Autodesk Inventor part; units mm, degrees
ref_plane "YZ Plane" through (0, 0, 0) normal (1, 0, 0) x (0, 1, 0)
ref_plane "XZ Plane" through (0, 0, 0) normal (0, 1, 0) x (-1, 0, 0)
ref_plane "XY Plane" through (0, 0, 0) normal (0, 0, 1) x (1, 0, 0)
sketch "Skizze1" plane through (0, 0, 0) normal (0, 1, 0) x (-1, 0, 0)
  line L0 (2.5, -1.4434) -> (0, -2.8868)
  line L1 (0, -2.8868) -> (-2.5, -1.4434)
  line L2 (-2.5, -1.4434) -> (-2.5, 1.4434)
  line L3 (-2.5, 1.4434) -> (0, 2.8868)
  line L4 (0, 2.8868) -> (2.5, 1.4434)
  line L5 (2.5, 1.4434) -> (2.5, -1.4434)
  point P0 (0, 0)
  point P1 (0, 0)
  point P2 (0, 0)
  dimension "d0" = 5
extrude "Extrusion1" add sketch "Skizze1" against normal blind 17
hole "Bohrung1" at (0, 0, 0) direction (0, -1, 0) diameter 2.013 depth 8 tip angle 118
sketch "Skizze2" plane through (0, -17, 0) normal (0, -1, 0) x (1, 0, 0)
  circle A0 centre (0, 0) radius 1.0065
  circle A1 centre (0, 0) radius 1.25
  dimension "d10" = 2.5
extrude "Extrusion2" add sketch "Skizze2" along normal blind 6 contours A0 | A1
thread "Gewinde1"
chamfer "Fasen1" distance 0.25 angle 45 1 edges at (-1.25, -23, 0)
chamfer "Fasen2" distance 0.3 angle 45 12 edges at (2.5, 0, 0) (1.25, 0, 2.1651) (-1.25, 0, 2.1651) (-2.5, 0, 0) (-1.25, 0, -2.1651) (1.25, 0, -2.1651) (2.5, -17, 0) (1.25, -17, 2.1651) (-1.25, -17, 2.1651) (-2.5, -17, 0) (-1.25, -17, -2.1651) (1.25, -17, -2.1651)
properties part number "Abstandsbolzen 17mm"
Work out the finished part from the listing and answer in its coordinate system (mm). A direction names the side the tool comes from. Give positions to 0.01 mm unless a question says otherwise; leave off trailing zeros. Loops run counter-clockwise (first coordinate to the right, second up) from the corner with the lowest first, then second, coordinate; pieces in that order, holes last. Notation, with made-up numbers: (11.25, 35) - (51.25, 35) arc R17 cw to (51.25, 66) - close; hole circle Ø8 at (14.25, 19.5). An arc over 180 degrees is marked (long way). Use CSV: the item, a comma, the result in double quotes. Start each with the question number.
(1) Find section D-D, the plane z = 2.3. Determine the outline of the cut face in (x, y).
(2) A tool of negligible diameter and unlimited length cuts with its end or side. For faces 5 (the face through (1, 0, -1)), 6 (the face through (-0.27, -19.83, 1.22)), from which of +Z, -Z, +X, -X, +Y, -Y can it reach the whole face along a straight path? Write none if from no direction.
(3) Find the intervals of material crossed by L1, parallel to X at y = -4.5, z = 0; L2, parallel to Y at x = 0.7, z = 1.6; L3, parallel to X at y = -2.75, z = 0.35, in increasing order.
(4) Find section B-B, the plane y = -10. Determine the outline of the cut face in (x, z), plus the area to 3 significant figures.
(5) Determine the mould class of faces 1 (the face through (1.233, -8.385, -2.175)), 2 (the face through (0.05, -8.5, 0.17)), 3 (the face through (-1.191, -0.148, -2.023)), 4 (the face through (1, -17, 1)) for opening direction X: released by +X, released by -X, zero draft, split by the parting line, or undercut.
(6) Each of these flat-tipped pins is pushed along its axis until it touches: pin 1 (1 mm diameter, centred on x = 1, y = -7, fed in from +Z); pin 2 (2 mm diameter, centred on x = -0.5, y = -10, fed in from -Z); pin 3 (3 mm diameter, centred on x = 2, y = -3.5, fed in from -Z). Where does it stop, or does it pass through?
(7) Find section A-A, the plane y = -2.5. Determine the outline of the cut face in (x, z), plus the area to 3 significant figures.
(8) Find section C-C, the plane x = -1.45. Determine the outline of the cut face in (y, z).
Results found:
1,outline,"(-1.02, -16.7) - (-0.42, -17) - (0.42, -17) - (1.02, -16.7) - (1.02, -0.3) - (0.42, 0) - (-0.42, 0) - (-1.02, -0.3) - close"
2,face 5,"+Z, -Z, +X, -X, +Y"
2,face 6,"-Y"
3,L1,"-2.5 to -1.01, 1.01 to 2.5"
3,L2,"-17 to 0"
3,L3,"-2.5 to -0.94, 0.94 to 2.5"
4,outline,"(-2.5, -1.44) - (0, -2.89) - (2.5, -1.44) - (2.5, 1.44) - (0, 2.89) - (-2.5, 1.44) - close"
4,area,"21.7 mm^2"
5,face 1,"released by +X"
5,face 2,"undercut"
5,face 3,"released by -X"
5,face 4,"zero draft"
6,pin 1,"z = 2.6"
6,pin 2,"z = -2.89"
6,pin 3,"z = -2.6"
7,outline,"(-2.5, -1.44) - (0, -2.89) - (2.5, -1.44) - (2.5, 1.44) - (0, 2.89) - (-2.5, 1.44) - close; hole circle Ø2.01 at (0, 0)"
7,area,"18.5 mm^2"
8,outline,"(-17, -1.7) - (-16.7, -2.05) - (-0.3, -2.05) - (0, -1.7) - (0, 1.7) - (-0.3, 2.05) - (-16.7, 2.05) - (-17, 1.7) - close"
